Geometry: final body of the model. Coordinates: model frame, mm. A direction names the side the tool comes from. Give positions to 0.01 mm unless a question says otherwise; leave off trailing zeros. Write each loop counter-clockwise with the first axis right and the second up, starting at its lowest first coordinate (ties: lowest second). Pieces come first, ordered by that corner, then holes. Notation, with made-up numbers: M -25,-7 L 29,-7 A21 cw 29,19 Z; hole C 17.25,43 d10. An arc over 180 degrees is marked long. Use one line per item in the form item = value. Start each with the question number.
Item 1: Material intervals for line 1 along X through (y, z) = (3.65, -0.85); line 2 along Z through (x, y) = (-2.25, 3.65); line 3 along Z through (x, y) = (-2, 0.65), sorted ascending. Write a range as from..to.
Item 2: Pull-direction query (X, two-part tool) for faces 3 (the flat face through (0, 3, 0)), 4 (the flat face through (5.2, 1.5, -0.4)), 5 (the flat face through (2, 3, -1.2)); classes: released by +X, released by -X, zero draft, split by the parting line, or undercut.
Item 3: Section query C-C on y = 0.5. Give the number of separate pieces and of enclosed holes in the cut face, then the cut area to 3 significant figures.
Item 4: Contact query for flat-ended pins moving along their axis: P1, Ø1, axis at x = 0.5, z = 1, coming from the -Y side; P2, Ø0.9, axis at x = 1.5, y = 3, coming from the +Z side. Output: stop coordinate, or through.
Item 5: Section query B-B on z = 0.6. Return loops of the section in (x, y), then the cut area to 3 significant figures.
Item 6: Access query for faces 1 (the flat face through (0.1, 0.5, 1.5)), 2 (the flat face through (-2.75, 3, -1)). Directions: +Z, -Z, +X, -X, +Y, -Y. A direction counts if a zero-diameter tool reaches every point of the face in a straight line with its end or side. Return the directions, or none.
Item 7: Section query A-A on y = 2.45. Return loops of the section in (x, z), then the cut area to 3 significant figures.
Autodesk Inventor part; units mm, degrees
ref_plane "YZ Plane" through (0, 0, 0) normal (1, 0, 0) x (0, 1, 0)
ref_plane "XZ Plane" through (0, 0, 0) normal (0, 1, 0) x (-1, 0, 0)
ref_plane "XY Plane" through (0, 0, 0) normal (0, 0, 1) x (1, 0, 0)
sketch "Sketch1" plane through (0, 0, 0) normal (0, 1, 0) x (-1, 0, 0)
  line L0 (5.2, -1.5) -> (-5.2, -1.5)
  line L1 (-5.2, -1.5) -> (-5.2, 1.5)
  line L2 (-5.2, 1.5) -> (5.2, 1.5)
  line L3 (5.2, 1.5) -> (5.2, -1.5)
  line L4 (7.28, 0) -> (-7.28, 0)
  line L5 (0, -2.1) -> (0, 2.1)
  point P0 (0, 0)
  dimension "d0" = 10.4
  dimension "d1" = 3
extrude "Extrusion1" add sketch "Sketch1" along normal blind 4
sketch "Sketch2" plane through (0, 4, 0) normal (0, 1, 0) x (1, 0, 0)
  line L0 (-5.2, -1.5) -> (5.2, -1.5)
  line L1 (5.2, -1.5) -> (5.2, 1.5)
  line L2 (-5.2, -1.5) -> (5.2, -1.5)
  line L3 (5.2, -1.5) -> (5.2, 0)
  line L4 (5.2, 0) -> (-5.2, 0)
  line L5 (-5.2, 0) -> (-5.2, -1.5)
  line L6 (-4.75, 0.3) -> (-3.25, 0.3)
  line L7 (-3.25, 0.3) -> (-3.25, 1.2)
  line L8 (-3.25, 1.2) -> (-4.75, 1.2)
  line L9 (-4.75, 1.2) -> (-4.75, 0.3)
  line L10 (-5.2, 1.5) -> (-5.2, -1.5)
  line L11 (-2.75, 0.3) -> (-1.25, 0.3)
  line L12 (-1.25, 0.3) -> (-1.25, 1.2)
  line L13 (-1.25, 1.2) -> (-2.75, 1.2)
  line L14 (-2.75, 1.2) -> (-2.75, 0.3)
  line L15 (-0.75, 0.3) -> (0.75, 0.3)
  line L16 (0.75, 0.3) -> (0.75, 1.2)
  line L17 (0.75, 1.2) -> (-0.75, 1.2)
  line L18 (-0.75, 1.2) -> (-0.75, 0.3)
  line L19 (1.25, 0.3) -> (2.75, 0.3)
  line L20 (2.75, 0.3) -> (2.75, 1.2)
  line L21 (2.75, 1.2) -> (1.25, 1.2)
  line L22 (1.25, 1.2) -> (1.25, 0.3)
  line L23 (3.25, 0.3) -> (4.75, 0.3)
  line L24 (4.75, 0.3) -> (4.75, 1.2)
  line L25 (4.75, 1.2) -> (3.25, 1.2)
  line L26 (3.25, 1.2) -> (3.25, 0.3)
  point P0 (0, 0)
  dimension "d4" = 1.5
  dimension "d5" = 0.9
  dimension "d6" = 0.3
  dimension "d7" = 0.45
  dimension "d10" = 2
extrude "Extrusion2" cut sketch "Sketch2" against normal blind 3
sketch "Sketch3" plane through (0, 1, 0) normal (0, 1, 0) x (1, 0, 0)
  line L0 (3.75, -0.9) -> (3.25, -0.9)
  line L1 (3.25, -0.9) -> (3.25, -0.7)
  line L2 (3.25, -0.7) -> (3.75, -0.7)
  line L3 (3.75, -0.7) -> (3.75, -0.9)
  line L4 (5.2, 1.5) -> (-5.2, 1.5)
  line L5 (5.2, -1.5) -> (-5.2, -1.5)
  line L6 (5.2, 0) -> (5.2, -1.5)
  line L7 (1.25, -0.9) -> (0.75, -0.9)
  line L8 (0.75, -0.9) -> (0.75, -0.7)
  line L9 (0.75, -0.7) -> (1.25, -0.7)
  line L10 (1.25, -0.7) -> (1.25, -0.9)
  line L11 (-0.75, -0.9) -> (-1.25, -0.9)
  line L12 (-1.25, -0.9) -> (-1.25, -0.7)
  line L13 (-1.25, -0.7) -> (-0.75, -0.7)
  line L14 (-0.75, -0.7) -> (-0.75, -0.9)
  line L15 (-3.25, -0.9) -> (-3.75, -0.9)
  line L16 (-3.75, -0.9) -> (-3.75, -0.7)
  line L17 (-3.75, -0.7) -> (-3.25, -0.7)
  line L18 (-3.25, -0.7) -> (-3.25, -0.9)
  line L19 (-5.2, -1.5) -> (-5.2, 0)
  line L20 (-3.75, 0.65) -> (-4.25, 0.65)
  line L21 (-4.25, 0.65) -> (-4.25, 0.85)
  line L22 (-4.25, 0.85) -> (-3.75, 0.85)
  line L23 (-3.75, 0.85) -> (-3.75, 0.65)
  line L24 (-4.75, 0.3) -> (-4.75, 1.2)
  line L25 (-3.25, 1.2) -> (-3.25, 0.3)
  line L26 (-4.75, 1.2) -> (-3.25, 1.2)
  line L27 (-3.25, 0.3) -> (-4.75, 0.3)
  line L28 (-1.75, 0.85) -> (-1.75, 0.65)
  line L29 (-1.75, 0.65) -> (-2.25, 0.65)
  line L30 (-2.25, 0.85) -> (-1.75, 0.85)
  line L31 (-2.25, 0.65) -> (-2.25, 0.85)
  line L32 (0.25, 0.85) -> (0.25, 0.65)
  line L33 (0.25, 0.65) -> (-0.25, 0.65)
  line L34 (-0.25, 0.85) -> (0.25, 0.85)
  line L35 (-0.25, 0.65) -> (-0.25, 0.85)
  line L36 (2.25, 0.85) -> (2.25, 0.65)
  line L37 (2.25, 0.65) -> (1.75, 0.65)
  line L38 (1.75, 0.85) -> (2.25, 0.85)
  line L39 (1.75, 0.65) -> (1.75, 0.85)
  line L40 (4.25, 0.85) -> (4.25, 0.65)
  line L41 (4.25, 0.65) -> (3.75, 0.65)
  line L42 (3.75, 0.85) -> (4.25, 0.85)
  line L43 (3.75, 0.65) -> (3.75, 0.85)
  point P0 (0, 0)
  dimension "d18" = 0.2
  dimension "d19" = 0.5
  dimension "d20" = 0.6
  dimension "d21" = 1.45
  dimension "d22" = 0.2
  dimension "d23" = 0.5
  dimension "d24" = 0.2
  dimension "d25" = 0.5
  dimension "d26" = 0.2
  dimension "d27" = 0.5
  dimension "d28" = 3.95
  dimension "d29" = 1.45
  dimension "d30" = 3.95
  dimension "d36" = 0.2
  dimension "d37" = 0.5
  dimension "d38" = 0.5
  dimension "d39" = 0.5
  dimension "d40" = 0.35
  dimension "d41" = 0.35
  dimension "d44" = 2
extrude "Extrusion3" cut sketch "Sketch3" against normal up to surface (1 mm away) contours L0 L1 L2 L3 | L7 L8 L9 L10 | L11 L12 L13 L14 | L15 L16 L17 L18 | L20 L21 L22 L23 | L28 L29 L31 L30 | L32 L33 L35 L34 | L36 L37 L39 L38 | L40 L41 L43 L42
chamfer "Chamfer1" distance 0.2 angle 45 36 edges at (-3.75, 1, 0.8) (-3.5, 1, 0.7) (-3.5, 1, 0.9) (-3.25, 1, 0.8) (-1.25, 1, 0.8) (-1, 1, 0.7) (-1, 1, 0.9) (-0.75, 1, 0.8) (0.75, 1, 0.8) (1, 1, 0.7) (1, 1, 0.9) (1.25, 1, 0.8) (3.25, 1, 0.8) (3.5, 1, 0.7) (3.5, 1, 0.9) (3.75, 1, 0.8) (3.75, 1, -0.75) (4, 1, -0.65) (4.25, 1, -0.75) (4, 1, -0.85) (2.25, 1, -0.75) (2, 1, -0.85) (1.75, 1, -0.75) (2, 1, -0.65) (0, 1, -0.65) (0.25, 1, -0.75) (-0.25, 1, -0.75) (0, 1, -0.85) (-1.75, 1, -0.75) (-2, 1, -0.85) (-2, 1, -0.65) (-2.25, 1, -0.75) (-3.75, 1, -0.75) (-4, 1, -0.85) (-4, 1, -0.65) (-4.25, 1, -0.75)
equation "\"d29\" = d21"
equation "\"d30\" = d28"
equation "\"d38\" = d39"
equation "\"d40\" = d41"
properties part number "USB 3.0 A Recepticle Rear Insert Fit" material "PBT Plastic"
Answer sheet:
q1.line_1 = -5.2..-4.75, -3.25..-2.75, -1.25..-0.75, 0.75..1.25, 2.75..3.25, 4.75..5.2
q1.line_2 = -1.5..-1.2, -0.3..0
q1.line_3 = -1.5..-0.85, -0.65..1.5
q2.face_3 = zero draft
q2.face_4 = released by +X
q2.face_5 = undercut
q3.separate_pieces = 1
q3.enclosed_holes = 9
q3.area = 30.3 mm2
q4.P1 = 0
q4.P2 = 0
q5.outline = M -5.2,0 L 5.2,0 L 5.2,1 L 3.95,1 L 3.85,0.9 L 3.15,0.9 L 3.05,1 L 1.45,1 L 1.35,0.9 L 0.65,0.9 L 0.55,1 L -0.55,1 L -0.65,0.9 L -1.35,0.9 L -1.45,1 L -3.05,1 L -3.15,0.9 L -3.85,0.9 L -3.95,1 L -5.2,1 Z
q5.area = 10.1 mm2
q6.face_1 = +Z, +X, -X, +Y, -Y
q6.face_2 = +Y
q7.outline = M -5.2,-1.5 L 5.2,-1.5 L 5.2,0 L -5.2,0 Z; hole M -4.75,-1.2 L -3.25,-1.2 L -3.25,-0.3 L -4.75,-0.3 Z; hole M -2.75,-1.2 L -1.25,-1.2 L -1.25,-0.3 L -2.75,-0.3 Z; hole M -0.75,-1.2 L 0.75,-1.2 L 0.75,-0.3 L -0.75,-0.3 Z; hole M 1.25,-1.2 L 2.75,-1.2 L 2.75,-0.3 L 1.25,-0.3 Z; hole M 3.25,-1.2 L 4.75,-1.2 L 4.75,-0.3 L 3.25,-0.3 Z
q7.area = 8.85 mm2
